The listing builds one solid part. Answer for the finished solid, in the listing's coordinates (mm). Coordinates: 2 decimals unless noted, no trailing zeros. Loops run counter-clockwise (first coordinate to the right, second up) from the corner with the lowest first, then second, coordinate; pieces in that order, holes last. Notation, with made-up numbers: (37.25, 7) -> (47.25, 7) arc R27 cw to (47.25, 44) -> close; hole circle Ø1 at (88.5, 66). An arc over 180 degrees is marked (long way). Answer in a Markdown table with one row per item.
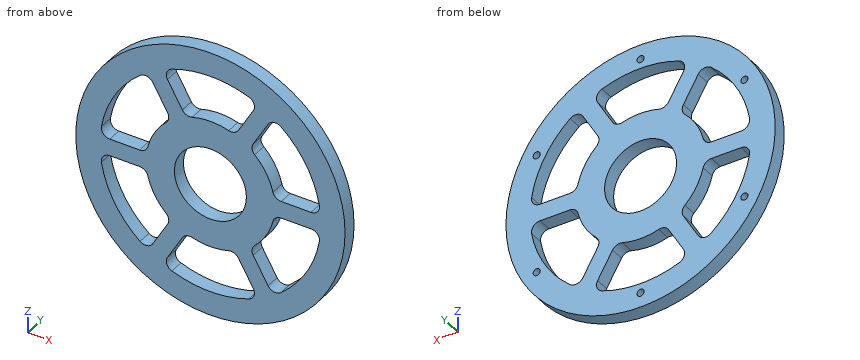
```python
from build123d import *

# Parameters (mm, degrees)
SKETCH1_R           = 47.5
BOSS_EXTRUDE1_DEPTH = 5
SKETCH2_R           = 12.7
CUT_EXTRUDE1_DEPTH  = 6
SKETCH3_R           = 1.25
CUT_EXTRUDE2_DEPTH  = 2.5
CUT_EXTRUDE3_DEPTH  = 6
FILLET1_R           = 3


with BuildPart() as part:
    # Sketch1 → Boss-Extrude1 (new body)
    with BuildSketch(Plane(origin=(0, 0, 0), x_dir=(1, 0, 0), z_dir=(0, 1, 0))):
        Circle(SKETCH1_R)
    extrude(amount=BOSS_EXTRUDE1_DEPTH)

    # Sketch2 → Cut-Extrude1 (cut, through all)
    with BuildSketch(Plane(origin=(0, 5, 0), x_dir=(1, 0, 0), z_dir=(0, 1, 0))):
        Circle(SKETCH2_R)
    extrude(amount=-CUT_EXTRUDE1_DEPTH, mode=Mode.SUBTRACT)

    # Sketch3 → Cut-Extrude2 (cut)
    with BuildSketch(Plane(origin=(0, 5, 0), x_dir=(1, 0, 0), z_dir=(0, 1, 0))):
        with Locations((0, 42.31)):
            Circle(SKETCH3_R)
        with Locations((36.641534834, 21.155)):
            Circle(SKETCH3_R)
        with Locations((36.641534834, -21.155)):
            Circle(SKETCH3_R)
        with Locations((0, -42.31)):
            Circle(SKETCH3_R)
        with Locations((-36.641534834, -21.155)):
            Circle(SKETCH3_R)
        with Locations((-36.641534834, 21.155)):
            Circle(SKETCH3_R)
    extrude(amount=-CUT_EXTRUDE2_DEPTH, mode=Mode.SUBTRACT)

    # Sketch4 → Cut-Extrude3 (cut, through all)
    with BuildSketch(Plane(origin=(0, 5, 0), x_dir=(1, 0, 0), z_dir=(0, 1, 0))):
        with BuildLine():
            Line((-13.848520647, 17.98634137), (-22.040298307, 32.174916481))
            ThreePointArc((-22.040298307, 32.174916481), (-33.774990748, 19.5), (-38.88444419, 3))
            Line((-38.88444419, 3), (-22.500888871, 3))
            ThreePointArc((-22.500888871, 3), (-19.658776666, 11.35), (-13.848520647, 17.98634137))
        make_face()
        with BuildLine():
            ThreePointArc((16.844145884, 35.174916481), (0, 39), (-16.844145884, 35.174916481))
            Line((-16.844145884, 35.174916481), (-8.652368224, 20.98634137))
            ThreePointArc((-8.652368224, 20.98634137), (0, 22.7), (8.652368224, 20.98634137))
            Line((8.652368224, 20.98634137), (16.844145884, 35.174916481))
        make_face()
        with BuildLine():
            ThreePointArc((38.88444419, 3), (33.774990748, 19.5), (22.040298307, 32.174916481))
            Line((22.040298307, 32.174916481), (13.848520647, 17.98634137))
            ThreePointArc((13.848520647, 17.98634137), (19.658776666, 11.35), (22.500888871, 3))
            Line((22.500888871, 3), (38.88444419, 3))
        make_face()
        with BuildLine():
            ThreePointArc((22.040298307, -32.174916481), (33.774990748, -19.5), (38.88444419, -3))
            Line((38.88444419, -3), (22.500888871, -3))
            ThreePointArc((22.500888871, -3), (19.658776666, -11.35), (13.848520647, -17.98634137))
            Line((13.848520647, -17.98634137), (22.040298307, -32.174916481))
        make_face()
        with BuildLine():
            Line((-8.652368224, -20.98634137), (-16.844145884, -35.174916481))
            ThreePointArc((-16.844145884, -35.174916481), (0, -39), (16.844145884, -35.174916481))
            Line((16.844145884, -35.174916481), (8.652368224, -20.98634137))
            ThreePointArc((8.652368224, -20.98634137), (0, -22.7), (-8.652368224, -20.98634137))
        make_face()
        with BuildLine():
            Line((-22.500888871, -3), (-38.88444419, -3))
            ThreePointArc((-38.88444419, -3), (-33.774990748, -19.5), (-22.040298307, -32.174916481))
            Line((-22.040298307, -32.174916481), (-13.848520647, -17.98634137))
            ThreePointArc((-13.848520647, -17.98634137), (-19.658776666, -11.35), (-22.500888871, -3))
        make_face()
    extrude(amount=-CUT_EXTRUDE3_DEPTH, mode=Mode.SUBTRACT)

    # Fillet1
    fillet1_edges = [part.edges().sort_by_distance(p)[0] for p in [
        (22.500888871, 2.5, -3),
        (13.848520647, 2.5, -17.98634137),
        (22.040298307, 2.5, -32.174916481),
        (38.88444419, 2.5, -3),
        (8.652368224, 2.5, -20.98634137),
        (-8.652368224, 2.5, -20.98634137),
        (-16.844145884, 2.5, -35.174916481),
        (16.844145884, 2.5, -35.174916481),
        (-8.652368224, 2.5, 20.98634137),
        (8.652368224, 2.5, 20.98634137),
        (16.844145884, 2.5, 35.174916481),
        (-16.844145884, 2.5, 35.174916481),
        (13.848520647, 2.5, 17.98634137),
        (22.500888871, 2.5, 3),
        (38.88444419, 2.5, 3),
        (22.040298307, 2.5, 32.174916481),
        (-22.500888871, 2.5, 3),
        (-13.848520647, 2.5, 17.98634137),
        (-22.040298307, 2.5, 32.174916481),
        (-38.88444419, 2.5, 3),
        (-13.848520647, 2.5, -17.98634137),
        (-22.500888871, 2.5, -3),
        (-38.88444419, 2.5, -3),
        (-22.040298307, 2.5, -32.174916481),
    ]]
    fillet(fillet1_edges, radius=FILLET1_R)


solid = part.part
```
Item 1: A cutting plane is placed at C-C, the plane x = 29. Determine the outline of the cut face in (y, z).
Findings below:
| item | result |
|---|---|
| outline | (0, -37.62) -> (5, -37.62) -> (5, -26.08) -> (0, -26.08) -> close; (0, -3) -> (5, -3) -> (5, 3) -> (0, 3) -> close; (0, 26.08) -> (5, 26.08) -> (5, 37.62) -> (0, 37.62) -> close |
Item 2: A cutting plane is placed at A-A, the plane x = 0. Determine the outline of the cut face in (y, z), plus the area to 4 significant figures.
Findings below:
| item | result |
|---|---|
| outline | (0, -47.5) -> (5, -47.5) -> (5, -43.56) -> (2.5, -43.56) -> (2.5, -41.06) -> (5, -41.06) -> (5, -39) -> (0, -39) -> close; (0, -22.7) -> (5, -22.7) -> (5, -12.7) -> (0, -12.7) -> close; (0, 12.7) -> (5, 12.7) -> (5, 22.7) -> (0, 22.7) -> close; (0, 39) -> (5, 39) -> (5, 41.06) -> (2.5, 41.06) -> (2.5, 43.56) -> (5, 43.56) -> (5, 47.5) -> (0, 47.5) -> close |
| area | 172.5 mm2 |
Item 3: A cutting plane is placed at B-B, the plane z = 0. Determine the outline of the cut face in (x, y).
Findings below:
| item | result |
|---|---|
| outline | (-47.5, 0) -> (-12.7, 0) -> (-12.7, 5) -> (-47.5, 5) -> close; (12.7, 0) -> (47.5, 0) -> (47.5, 5) -> (12.7, 5) -> close |
Item 4: A cutting plane is placed at D-D, the plane z = -42.31. Determine the outline of the cut face in (x, y), plus the area to 3 significant figures.
Findings below:
| item | result |
|---|---|
| outline | (-21.59, 0) -> (21.59, 0) -> (21.59, 5) -> (1.25, 5) -> (1.25, 2.5) -> (-1.25, 2.5) -> (-1.25, 5) -> (-21.59, 5) -> close |
| area | 210 mm2 |
Item 5: Flat-ended cylindrical pins translate along their axes: pin 1 Ø3 at (y, z) = (2, -28.5) entering from +X; pin 2 Ø2.5 at (x, y) = (-28.5, 3.5) entering from -Z; pin 3 Ø20.5 at (x, z) = (0, 0) entering from +Y; pin 4 Ø1 at (x, y) = (1, 4) entering from -Z. Find the tip coordinate at first contact, or state that the pin passes through.
Findings below:
| item | result |
|---|---|
| pin 1 | stops at x = 39.08 |
| pin 2 | stops at z = -38.91 |
| pin 3 | passes through |
| pin 4 | stops at z = -47.5 |
Item 6: Find the intervals of material crossed by probe 1 along X at (y, z) = (2.05, -18); probe 2 along X at (y, z) = (3.4, -30.5); probe 3 along X at (y, z) = (1.6, 5.5), in increasing order.
Findings below:
| item | result |
|---|---|
| probe 1 | x = -43.96 to -34.6, -14.76 to 14.76, 34.6 to 43.96 |
| probe 2 | x = -36.41 to -24.12, -21.77 to -14.15, 14.15 to 21.77, 24.12 to 36.41 |
| probe 3 | x = -47.18 to -38.45, -22.02 to -11.45, 11.45 to 22.02, 38.45 to 47.18 |
